Design review of the part shown in the three views and the two pictorial views. Dimensions are in mm from the part's minimum x, y and z. Coordinates: 2 decimals unless noted, no trailing zeros. Write each loop counter-clockwise with the first axis right and the second up, starting at its lowest first coordinate (ties: lowest second). Pieces come first, ordered by that corner, then holes. Notation, with made-up numbers: (15, 29) -> (49, 29) arc R18 cw to (49, 40) -> close; hole circle Ø2 at (13, 61.5). An arc over 180 degrees is marked (long way). Answer in a Markdown table with one row per item. Add a question column.
Item 1: Take a section at C-C, the plane z = 10. Write out the cut boundary in (x, y).
Item 2: Take a section at A-A, the plane x = 10. Write out the cut boundary in (y, z), and give its area (3 significant figures).
Item 3: Take a section at D-D, the plane x = 110. Write out the cut boundary in (y, z).
Item 4: Take a section at B-B, the plane y = 1.35. Write out the cut boundary in (x, z).
Item 5: To check wall thickness, follow line 1 (Z direction, x = 10, y = 4.4); line 2 (X direction, y = 4.95, z = 29); line 3 (X direction, y = 3.7, z = 32). State the ranges of each line that lie inside material, in increasing order.
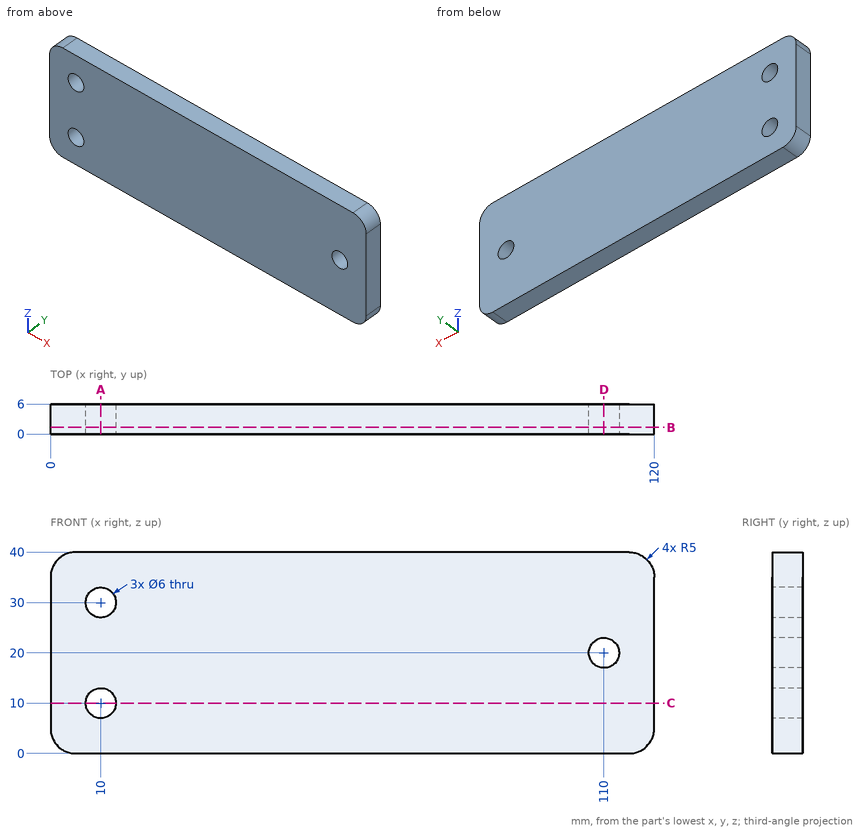
Answers:
| question | item | result |
|---|---|---|
| 1 | outline | (0, 0) -> (7, 0) -> (7, 6) -> (0, 6) -> close; (13, 0) -> (120, 0) -> (120, 6) -> (13, 6) -> close |
| 2 | outline | (0, 0) -> (6, 0) -> (6, 7) -> (0, 7) -> close; (0, 13) -> (6, 13) -> (6, 27) -> (0, 27) -> close; (0, 33) -> (6, 33) -> (6, 40) -> (0, 40) -> close |
| 2 | area | 168 mm^2 |
| 3 | outline | (0, 0) -> (6, 0) -> (6, 17) -> (0, 17) -> close; (0, 23) -> (6, 23) -> (6, 40) -> (0, 40) -> close |
| 4 | outline | (0, 5) arc R5 ccw to (5, 0) -> (115, 0) arc R5 ccw to (120, 5) -> (120, 35) arc R5 ccw to (115, 40) -> (5, 40) arc R5 ccw to (0, 35) -> close; hole circle Ø6 at (10, 10); hole circle Ø6 at (10, 30); hole circle Ø6 at (110, 20) |
| 5 | line 1 | z = 0 to 7, 13 to 27, 33 to 40 |
| 5 | line 2 | x = 0 to 7.17, 12.83 to 120 |
| 5 | line 3 | x = 0 to 7.76, 12.24 to 120 |
